Study the drawing (mm; zero at the part's minimum x, y, z) and answer. A direction names the side the tool comes from. Give positions to 0.01 mm unless a question says otherwise; leave off trailing zeros. Write each loop counter-clockwise with the first axis right and the second up, starting at its lowest first coordinate (ties: lowest second). Pieces come first, ordered by that corner, then holes. Notation, with made-up numbers: M 61.5,71.5 L 97.5,71.5 A20 ccw 97.5,101.5 Z; hole C 89.5,-1.75 d10. An arc over 180 degrees is marked long. Use a Markdown table: item, result. Add a question column.
Item 1: A cutting plane is placed at A-A on z = 5.45. Determine the outline of the cut face in (x, y).
Item 2: A cutting plane is placed at D-D on z = 9.5. Determine the outline of the cut face in (x, y).
Item 3: The mould has two halves that part along X. Classify the marked faces 3, 4, 5 and 6: pulls with the +X half, pulls with the -X half, needs draft (parallel to the pull), parting line crosses it, or undercut.
Item 4: A cutting plane is placed at C-C on x = 2.7. Determine the outline of the cut face in (y, z) (3 decimals), then the cut area to 3 significant figures.
Item 5: Consider probe 1 along X at (y, z) = (2.25, 5.45); probe 2 along Y at (x, z) = (1.5, 8.75); probe 3 along Z at (x, y) = (2.25, 19.25). Determine where each line is inside the solid, lowest interval first. Write a range as [from, to].
Item 6: For the marked faces 1 and 2, determine the directions among +Z, -Z, +X, -X, +Y, -Y from which every point of the face is accessible in a straight line to the end or side of a thin tool.
Item 7: A cutting plane is placed at B-B on y = 18.75. Determine the outline of the cut face in (x, z).
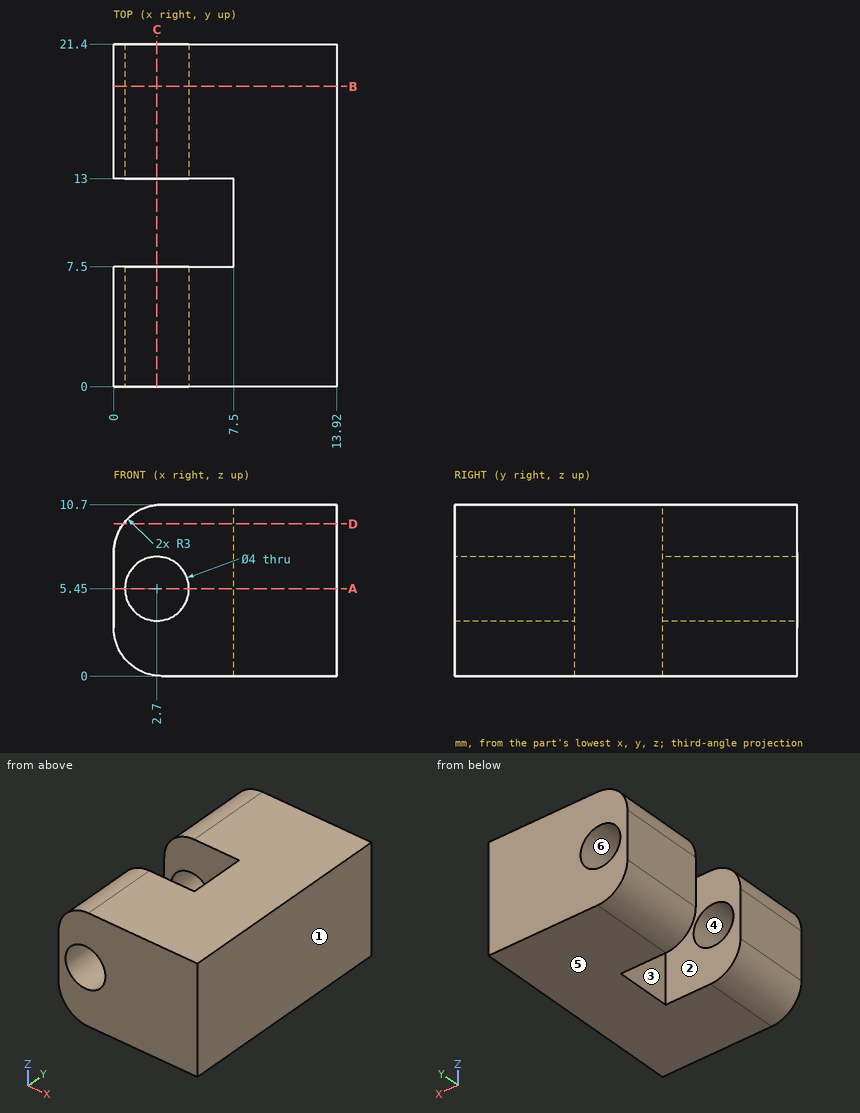
Filled in:
| question | item | result |
|---|---|---|
| 1 | outline | M 0,0 L 0.7,0 L 0.7,7.5 L 0,7.5 Z; M 0,13 L 0.7,13 L 0.7,21.4 L 0,21.4 Z; M 4.7,0 L 13.92,0 L 13.92,21.4 L 4.7,21.4 L 4.7,13 L 7.5,13 L 7.5,7.5 L 4.7,7.5 Z |
| 2 | outline | M 0.6,0 L 13.92,0 L 13.92,21.4 L 0.6,21.4 L 0.6,13 L 7.5,13 L 7.5,7.5 L 0.6,7.5 Z |
| 3 | face 3 | pulls with the -X half |
| 3 | face 4 | undercut |
| 3 | face 5 | needs draft |
| 3 | face 6 | undercut |
| 4 | outline | M 0,0.015 L 7.5,0.015 L 7.5,3.45 L 0,3.45 Z; M 0,7.45 L 7.5,7.45 L 7.5,10.685 L 0,10.685 Z; M 13,0.015 L 21.4,0.015 L 21.4,3.45 L 13,3.45 Z; M 13,7.45 L 21.4,7.45 L 21.4,10.685 L 13,10.685 Z |
| 4 | area | 106 mm² |
| 5 | probe 1 | [0, 0.7], [4.7, 13.92] |
| 5 | probe 2 | [0, 7.5], [13, 21.4] |
| 5 | probe 3 | [0.1, 3.5], [7.4, 10.6] |
| 6 | face 1 | +Z, -Z, +X, +Y, -Y |
| 6 | face 2 | +Z, -Z, -X |
| 7 | outline | M 0,3 A3 ccw 3,0 L 13.92,0 L 13.92,10.7 L 3,10.7 A3 ccw 0,7.7 Z; hole C 2.7,5.45 d4 |
